from build123d import *

# Parameters (mm, degrees)
SKETCH_R     = 2.5
SKETCH_R_2   = 1.5
PAD_DEPTH    = 13
POCKET_DEPTH = 2.5


with BuildPart() as part:
    # Sketch → Pad (new body)
    with BuildSketch(Plane.XY):
        Circle(SKETCH_R)
        Circle(SKETCH_R_2, mode=Mode.SUBTRACT)
    extrude(amount=PAD_DEPTH)

    # Sketch001 (on DatumPlane) → Pocket (cut)
    with BuildSketch(Plane.YZ.offset(2.5)):
        with BuildLine():
            ThreePointArc((1.5, 4.5), (0, 6), (-1.5, 4.5))
            Line((-1.5, 4.5), (-1.5, 2.5))
            ThreePointArc((-1.5, 2.5), (0, 1), (1.5, 2.5))
            Line((1.5, 4.5), (1.5, 2.5))
        make_face()
    extrude(amount=-POCKET_DEPTH, mode=Mode.SUBTRACT)


solid = part.part
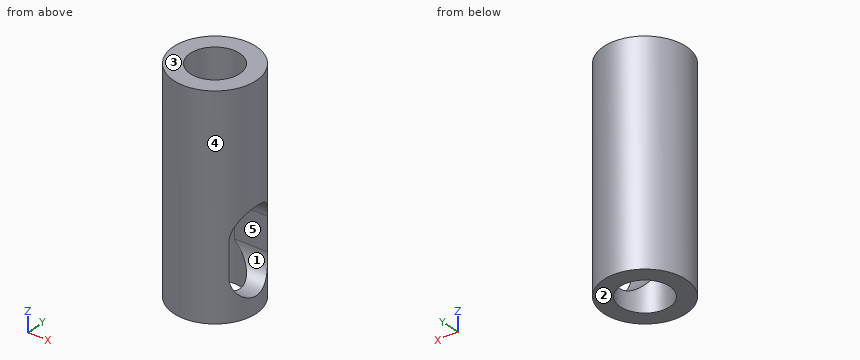
Part model, mm, in its own coordinate system. Face numbers are marked on the shaded views. A direction names the side the tool comes from. Coordinates: 2 decimals unless noted, no trailing zeros. Loops run counter-clockwise (first coordinate to the right, second up) from the corner with the lowest first, then second, coordinate; pieces in that order, holes last. Notation, with made-up numbers: M 50,59 L 100,59 A22 cw 100,98 Z; hole C 35,69.5 d3. An arc over 180 degrees is marked long. Use a Markdown table: item, result. Add a question column.
Q1. Pin check, flat tips, straight feed: P1, Ø1, axis at x = 1, z = 4.5, coming from the -Y side; P2, Ø1.6, axis at x = 0.5, z = 3.5, coming from the +Y side; P3, Ø1.5, axis at x = 2, z = 9, coming from the +Y side. Stop position of each tip, or through.
Q2. Which spindle directions (+Z, -Z, +X, -X, +Y, -Y) get a long thin tool onto all of the face, cutting with end or side? Do the marked faces 1 and 2. Say none if no direction does.
Q3. Mould opens along Y. For the marked faces 3, 4 and 5 say: +Y half, -Y half, draft (parallel to the pull), parting line (faces both ways), or undercut.
Q4. Cut at C-C (z = 10.25). Write the cut outline in (x, y), and give its area (3 significant figures).
Q5. Probe L1, parallel to Y at x = 0, z = 5.75; L2, parallel to Y at x = 0.4, z = 5.5; L3, parallel to X at y = -1.15, z = 6.75. List the from-to ranges inside material, lowest first.
Q6. Cut at B-B (x = 0.7). Write the cut outline in (y, z), and give its area (3 significant figures).
Q7. Cut at D-D (y = 1.2). Write the cut outline in (x, z), and give its area (3 significant figures).
Q8. Cut at A-A (y = 0). Write the cut outline in (x, z), and give its area (3 significant figures).
Worked out:
| question | item | result |
|---|---|---|
| 1 | P1 | stops at y = -2.45 |
| 1 | P2 | stops at y = 2.5 |
| 1 | P3 | stops at y = 2.17 |
| 2 | face 1 | +X |
| 2 | face 2 | -Z, +X, -X, +Y, -Y |
| 3 | face 3 | draft |
| 3 | face 4 | parting line |
| 3 | face 5 | undercut |
| 4 | outline | C 0,0 d5; hole C 0,0 d3 |
| 4 | area | 12.6 mm2 |
| 5 | L1 | y = -2.5 to -1.5, 1.5 to 2.5 |
| 5 | L2 | y = -2.47 to -1.45, 1.45 to 2.47 |
| 5 | L3 | x = -2.22 to -0.96, 0.96 to 2.22 |
| 6 | outline | M -2.4,0 L -1.33,0 L -1.33,1.8 A1.5 cw -1.5,2.5 L -1.5,4.5 A1.5 cw -1.33,5.2 L -1.33,13 L -2.4,13 Z; M 1.33,0 L 2.4,0 L 2.4,13 L 1.33,13 L 1.33,5.2 A1.5 cw 1.5,4.5 L 1.5,2.5 A1.5 cw 1.33,1.8 Z |
| 6 | area | 26.9 mm2 |
| 7 | outline | M -2.19,0 L -0.9,0 L -0.9,13 L -2.19,13 Z; M 0.9,0 L 2.19,0 L 2.19,1.6 L 0.9,1.6 Z; M 0.9,5.4 L 2.19,5.4 L 2.19,13 L 0.9,13 Z |
| 7 | area | 28.7 mm2 |
| 8 | outline | M -2.5,0 L -1.5,0 L -1.5,13 L -2.5,13 Z; M 1.5,0 L 2.5,0 L 2.5,1 L 1.5,1 Z; M 1.5,6 L 2.5,6 L 2.5,13 L 1.5,13 Z |
| 8 | area | 21.0 mm2 |
